Verification items for the finished model (mm, model axes). Round coordinates to 2 decimals unless told otherwise and drop trailing zeros. Order: outer loops, then holes, each group sorted by start corner. A loop starts at its lowest first (then second) coordinate and runs counter-clockwise, first axis right, second up. Notation, with made-up numbers: M -6.5,-15.5 L 36.5,-15.5 A27 ccw 36.5,18.5 Z; hole C 42.5,-2 d11. An arc over 180 degrees is marked long. Write item = value, one per line. Start each with the question number.
from build123d import *

# Parameters (mm, degrees)
SKETCH_R           = 34
SKETCH_R_2         = 6.5
PAD_DEPTH          = 5
SKETCH001_R        = 1.5
POCKET_DEPTH       = 10
POLARPATTERN_COUNT = 6


with BuildPart() as part:
    # Sketch → Pad (new body)
    with BuildSketch(Plane.XY):
        Circle(SKETCH_R)
        Circle(SKETCH_R_2, mode=Mode.SUBTRACT)
    extrude(amount=PAD_DEPTH)

    # Sketch001 (on Face4 of Pad) → Pocket (cut)
    with BuildSketch(Plane.XY.offset(5)):
        with Locations((0, 22)):
            Circle(SKETCH001_R)
    pocket = extrude(amount=-POCKET_DEPTH, mode=Mode.SUBTRACT)

    # PolarPattern: Pocket ×6 about axis
    polarpattern_axis = Axis((0, 0, 5), (0, 0, 1))
    for i in range(1, POLARPATTERN_COUNT):
        add(pocket.rotate(polarpattern_axis, i * 360 / POLARPATTERN_COUNT), mode=Mode.SUBTRACT)


solid = part.part
1) Scan lines: probe 1 along Y at (x, z) = (0, 3.45); probe 2 along Y at (x, z) = (-19.5, 3.6); probe 3 along X at (y, z) = (4, 2.25). Record each from-to range of solid material in increasing order.
2) Cross-section at D-D, the plane y = -11. Enter the section's corners in (x, z), then the cut area to 3 significant figures.
3) Cross-section at C-C, the plane z = 1.05. Enter the section's corners in (x, y), then the cut area to 3 significant figures.
4) Cross-section at A-A, the plane y = 0. Enter the section's corners in (x, z), then the cut area to 3 significant figures.
5) Cross-section at B-B, the plane x = 0. Enter the section's corners in (y, z), then the cut area to 3 significant figures.
6) Release check for a two-part mould opening along X. For faces 1 (the flat face through (0, -7, 0)), 2 (the cylindrical face through (17.667, 11.575, 2.535)), 3 (the cylindrical face through (18.28, 28.67, 2.46)), 4 (the cylindrical face through (0.195, -23.487, 2.535)) record: pulls with the +X half, pulls with the -X half, needs draft (parallel to the pull), parting line crosses it, or undercut.
7) Gauge pin test, flat ends, axial feed: P1, Ø2.5, axis at x = -19.05, y = -11, coming from the +Z side; P2, Ø1, axis at y = -21, z = 3, coming from the -X side; P3, Ø1, axis at y = 19.5, z = 0.5, coming from the -X side; P4, Ø2, axis at y = -21, z = 1, coming from the -X side. Record the tip position at first contact, or that the pin passes through.
Geometry results:
q1.probe_1 = -34 to -23.5, -20.5 to -6.5, 6.5 to 20.5, 23.5 to 34
q1.probe_2 = -27.85 to -12.43, -9.57 to 9.57, 12.43 to 27.85
q1.probe_3 = -33.76 to -5.12, 5.12 to 33.76
q2.outline = M -32.17,0 L -20.55,0 L -20.55,5 L -32.17,5 Z; M -17.55,0 L 17.55,0 L 17.55,5 L -17.55,5 Z; M 20.55,0 L 32.17,0 L 32.17,5 L 20.55,5 Z
q2.area = 292 mm^2
q3.outline = C 0,0 d68; hole C -19.05,-11 d3; hole C -19.05,11 d3; hole C 0,0 d13; hole C 0,-22 d3; hole C 0,22 d3; hole C 19.05,-11 d3; hole C 19.05,11 d3
q3.area = 3,460 mm^2
q4.outline = M -34,0 L -6.5,0 L -6.5,5 L -34,5 Z; M 6.5,0 L 34,0 L 34,5 L 6.5,5 Z
q4.area = 275 mm^2
q5.outline = M -34,0 L -23.5,0 L -23.5,5 L -34,5 Z; M -20.5,0 L -6.5,0 L -6.5,5 L -20.5,5 Z; M 6.5,0 L 20.5,0 L 20.5,5 L 6.5,5 Z; M 23.5,0 L 34,0 L 34,5 L 23.5,5 Z
q5.area = 245 mm^2
q6.face_1 = needs draft
q6.face_2 = undercut
q6.face_3 = parting line crosses it
q6.face_4 = undercut
q7.P1 = through
q7.P2 = -27.12
q7.P3 = -28.2
q7.P4 = -27.5
